from build123d import *

# Parameters (mm, degrees)
F0_W     = 63.4514391422
F0_H     = 32.6035022736
F1_DEPTH = 25
F2_SIZE  = 12
F4_D     = 4.2
F5_SIZE  = 2


with BuildPart() as f1:
    # F0 (on Top) → F1 (new body)
    with BuildSketch(Plane.XY):
        with Locations((31.7257195711, 16.3017511368)):
            Rectangle(F0_W, F0_H)
    extrude(amount=F1_DEPTH)

    # F2
    f2_edges = [f1.edges().sort_by_distance(p)[0] for p in [
        (31.72572, 32.603502, 25),
    ]]
    chamfer(f2_edges, length=F2_SIZE)

    # F4 (through all)
    with Locations(Plane(origin=(0, 22.8017511368, 22.8017511368), x_dir=(-1, 0, 0), z_dir=(0, 0.7071067812, 0.7071067812))):
        with Locations((-12.4934799969, -4.4305082411), (-40.9099496901, -4.4305082411)):
            Hole(F4_D / 2)

    # F5
    f5_edges = [f1.edges().sort_by_distance(p)[0] for p in [
        (31.72572, 32.603502, 0),
    ]]
    chamfer(f5_edges, length=F5_SIZE)


solid = f1.part
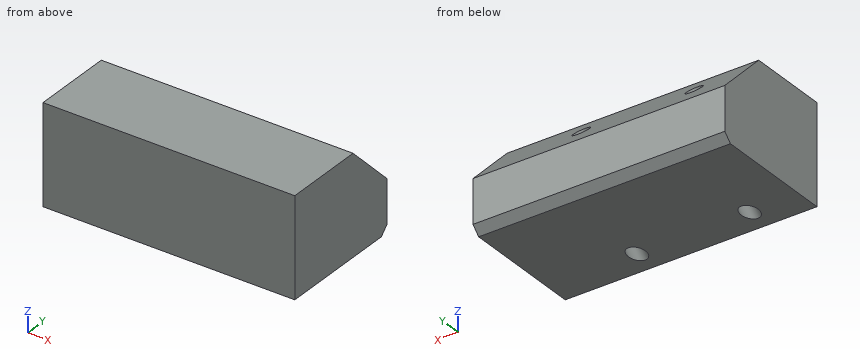
Work out the finished part from the listing and answer in its coordinate system (mm). Give positions to 0.01 mm unless a question says otherwise; leave off trailing zeros. Write each loop counter-clockwise with the first axis right and the second up, starting at its lowest first coordinate (ties: lowest second). Pieces come first, ordered by that corner, then holes.
Q1. The part is cut by section B-B on x = 42. Give the vertices of the cut face in (y, z).
Answer:
outline: (0, 0) - (3.73, 0) - (24.67, 20.94) - (20.6, 25) - (0, 25) - close; (8.8, 0) - (30.6, 0) - (32.6, 2) - (32.6, 13) - (27.2, 18.4) - close
Q2. The part is cut by section C-C on z = 14.75. State how many separate pieces and enclosed holes the cut face has, and give its area (3 significant figures).
Answer:
separate pieces: 1
enclosed holes: 2
area: 1,920 mm2
Q3. Straight lines are drawn through the part: L1, parallel to X at y = 13.5, z = 8.5; L2, parallel to X at y = 8, z = 3.5; L3, parallel to Y at x = 14, z = 16.25. For each, find the intervals that lie inside material, in ascending order.
Answer:
L1: x = 0 to 10.59, 14.39 to 39.01, 42.81 to 63.45
L2: x = 0 to 10.8, 14.18 to 39.22, 42.6 to 63.45
L3: y = 0 to 20.45, 24.58 to 29.35
Q4. The part is cut by section A-A on x = 52.5. Give the vertices of the cut face in (y, z), and give its area (3 significant figures).
Answer:
outline: (0, 0) - (30.6, 0) - (32.6, 2) - (32.6, 13) - (20.6, 25) - (0, 25) - close
area: 741 mm2
Q5. Given pin 1 (5 mm diameter, centred on x = 52.5, y = 27.5, fed in from +Z); pin 2 (4 mm diameter, centred on x = 18, y = 24, fed in from +Z); pin 3 (1.5 mm diameter, centred on x = 49, y = 23.5, fed in from +Z), each flat-ended and moving along its own axis, determine where each tip first touches the part or whether it passes through.
Answer:
pin 1: stops at z = 20.6
pin 2: stops at z = 23.6
pin 3: stops at z = 22.85
